```python
from build123d import *

# Parameters (mm, degrees)
SKETCH1_R      = 2.921
EXTRUDE1_DEPTH = 38.1
CHAMFER1_SIZE  = 0.5842
EXTRUDE7_DEPTH = 26.4


with BuildPart() as part:
    # Sketch1 → Extrude1 (new body, symmetric)
    with BuildSketch(Plane.XY):
        Circle(SKETCH1_R)
    extrude(amount=EXTRUDE1_DEPTH, both=True)

    # Chamfer1
    chamfer1_edges = [part.edges().sort_by_distance(p)[0] for p in [
        (-2.921, 0, -38.1),
        (-2.921, 0, 38.1),
    ]]
    chamfer(chamfer1_edges, length=CHAMFER1_SIZE)

    # Sketch13 → Extrude7 (cut, through all)
    with BuildSketch(Plane.XY.offset(12.7)):
        with BuildLine():
            Line((-1.4605, 2.529660204), (1.4605, 2.529660204))
            ThreePointArc((1.4605, 2.529660204), (0, 2.921), (-1.4605, 2.529660204))
        make_face()
    extrude(amount=EXTRUDE7_DEPTH, mode=Mode.SUBTRACT)


solid = part.part
```
Design review of the part built by this model. Coordinates are the model's own, in mm. A direction names the side the tool comes from. Coordinates: 2 decimals unless noted, no trailing zeros. Order: outer loops, then holes, each group sorted by start corner. A loop starts at its lowest first (then second) coordinate and runs counter-clockwise, first axis right, second up. Notation, with made-up numbers: (46.5, 7) - (73.5, 7) arc R17 cw to (73.5, 40) - close; hole circle Ø2 at (47.5, 46). An arc over 180 degrees is marked (long way). Answer in a Markdown table with one row per item.
(1) For faces 1 (the flat face through (0, 0, -38.1)), 2 (the flat face through (0, 2.53, 25)), list the 3-axis set-ups (+Z, -Z, +X, -X, +Y, -Y) from which the entire face can be reached by the end or side of a thin tool; tool diameter is ignored.
Checked values:
| item | result |
|---|---|
| face 1 | -Z, +X, -X, +Y, -Y |
| face 2 | +Z, +X, -X, +Y |
(2) Wall thickness on line 1 along X through (y, z) = (0.15, -28); line 2 along Y through (x, z) = (-0.1, 20.5); line 3 along Y through (x, z) = (-1.05, 23): over which ranges is each line inside the solid? List them lowest first. Write a range as from..to.
Checked values:
| item | result |
|---|---|
| line 1 | -2.92..2.92 |
| line 2 | -2.92..2.53 |
| line 3 | -2.73..2.53 |
(3) Clearance check with flat-ended pins moving along their axes: pin 1 (2 mm diameter, centred on x = -2.5, z = -6.5, fed in from -Y); pin 2 (1.5 mm diameter, centred on x = -0.5, z = 31, fed in from +Y); pin 3 (1.5 mm diameter, centred on x = 2, z = -20.5, fed in from -Y). State where each tip first meets the part, or that it passes through.
Checked values:
| item | result |
|---|---|
| pin 1 | y = -2.51 |
| pin 2 | y = 2.53 |
| pin 3 | y = -2.64 |
(4) Consider section B-B on z = -29.5. State the section outline as (x, y) points, plus the area to 3 significant figures.
Checked values:
| item | result |
|---|---|
| outline | circle Ø5.84 at (0, 0) |
| area | 26.8 mm^2 |
(5) Consider section A-A on x = 0. State the section outline as (y, z) points, plus the area to 3 significant figures.
Checked values:
| item | result |
|---|---|
| outline | (-2.92, -37.52) - (-2.34, -38.1) - (2.34, -38.1) - (2.92, -37.52) - (2.92, 12.7) - (2.53, 12.7) - (2.53, 37.91) - (2.34, 38.1) - (-2.34, 38.1) - (-2.92, 37.52) - close |
| area | 435 mm^2 |
